The model under review builds one solid part; all positions refer to its coordinate system, in mm. Face numbers are marked on the shaded views. A direction names the side the tool comes from. Round coordinates to 2 decimals unless told otherwise and drop trailing zeros. Loops run counter-clockwise (first coordinate to the right, second up) from the corner with the lowest first, then second, coordinate; pieces in that order, holes last. Notation, with made-up numbers: (71, 57.25) -> (125, 57.25) arc R12 ccw to (125, 67.25) -> close; hole circle Ø6 at (37.5, 74.5). An arc over 180 degrees is marked (long way). Write each question's results on one line, items separated by ' | '. Start each with the question number.
Item 1: Clearance check with flat-ended pins moving along their axes: pin 1 Ø6 at (x, z) = (39, 6.5) entering from -Y; pin 2 Ø1.5 at (x, z) = (39.5, 7) entering from -Y; pin 3 Ø6 at (x, y) = (31.5, -16.5) entering from +Z. State where each tip first meets the part, or that it passes through.
Item 2: Tool access review of the marked faces 1, 2 and 3: name each direction out of +Z, -Z, +X, -X, +Y, -Y from which nothing blocks a thin tool from reaching the whole face with its end or side.
Item 3: We need section C-C (y = -39.13). Give the boundary of the cut face in (x, z), and give its area (3 significant figures).
Item 4: For L1, parallel to Y at x = 25.25, z = 6.1; L2, parallel to X at y = 16, z = 9; L3, parallel to Y at x = 30.87, z = 2.85, list the stretches that pass through material, from the lowest coordinate up. Write a range as from..to.
Item 5: Mouldability with a two-part tool opening along X and no side actions: class the marked faces 4, 5, 6 and 7 as pulls with the +X half, pulls with the -X half, needs draft (parallel to the pull), parting line crosses it, or undercut.
Item 6: We need section D-D (y = -24.13). Give the boundary of the cut face in (x, z).
Item 7: We need section B-B (z = 3.25). Give the boundary of the cut face in (x, y), and give its area (3 significant figures).
Item 8: We need section A-A (y = 24.13). Give the boundary of the cut face in (x, z).
from build123d import *

# Parameters (mm, degrees)
SKETCH_W     = 20
SKETCH_H     = 83.26
SKETCH_R     = 1.75
SKETCH_R_2   = 2.25
PAD_DEPTH    = 5
PAD001_DEPTH = 5


with BuildPart() as part:
    # Sketch → Pad (new body)
    with BuildSketch(Plane.XY):
        with Locations((30.87, -7.5)):
            Rectangle(SKETCH_W, SKETCH_H)
        with Locations((25.25, -24.13)):
            Circle(SKETCH_R, mode=Mode.SUBTRACT)
        with Locations((32.87, 24.13)):
            Circle(SKETCH_R, mode=Mode.SUBTRACT)
        with Locations((30.87, -39.13)):
            Circle(SKETCH_R_2, mode=Mode.SUBTRACT)
    extrude(amount=PAD_DEPTH)

    # Sketch001 → Pad001 (new body)
    with BuildSketch(Plane.XY.offset(5)):
        with BuildLine():
            Line((20.87, 34.13), (20.87, -29.13))
            Line((20.87, -29.13), (25.87, -29.13))
            Line((25.87, -29.13), (25.87, -28.081658))
            ThreePointArc((25.87, -20.178342), (21.25, -24.13), (25.87, -28.081658))
            Line((25.87, 34.13), (25.87, -20.178342))
            Line((20.87, 34.13), (25.87, 34.13))
        make_face()
        with BuildLine():
            Line((40.87, 34.13), (35.87, 34.13))
            Line((35.87, 34.13), (35.87, 26.775751))
            ThreePointArc((35.87, 21.484249), (36.87, 24.13), (35.87, 26.775751))
            Line((35.87, -29.13), (35.87, 21.484249))
            Line((35.87, -29.13), (40.87, -29.13))
            Line((40.87, -29.13), (40.87, 34.13))
        make_face()
    extrude(amount=PAD001_DEPTH)


solid = part.part
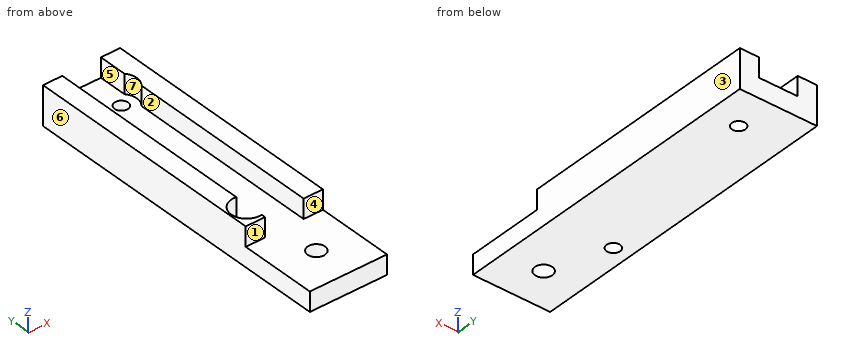
Here are the results:
1) pin 1: stops at y = -49.13 | pin 2: stops at y = -29.13 | pin 3: stops at z = 5
2) face 1: +Z, +X, -X, -Y | face 2: +Z, +Y, -Y | face 3: +Z, -Z, +X, +Y, -Y
3) outline: (20.87, 0) -> (28.62, 0) -> (28.62, 5) -> (20.87, 5) -> close; (33.12, 0) -> (40.87, 0) -> (40.87, 5) -> (33.12, 5) -> close | area: 77.5 mm2
4) L1: y = -29.13..-28.13, -20.13..34.13 | L2: x = 20.87..25.87, 35.87..40.87 | L3: y = -49.13..-41.38, -36.88..34.13
5) face 4: needs draft | face 5: undercut | face 6: pulls with the -X half | face 7: undercut
6) outline: (20.87, 0) -> (23.5, 0) -> (23.5, 5) -> (21.25, 5) -> (21.25, 10) -> (20.87, 10) -> close; (27, 0) -> (40.87, 0) -> (40.87, 10) -> (35.87, 10) -> (35.87, 5) -> (27, 5) -> close
7) outline: (20.87, -49.13) -> (40.87, -49.13) -> (40.87, 34.13) -> (20.87, 34.13) -> close; hole circle Ø3.5 at (25.25, -24.13); hole circle Ø4.5 at (30.87, -39.13); hole circle Ø3.5 at (32.87, 24.13) | area: 1,630 mm2
8) outline: (20.87, 0) -> (31.12, 0) -> (31.12, 5) -> (25.87, 5) -> (25.87, 10) -> (20.87, 10) -> close; (34.62, 0) -> (40.87, 0) -> (40.87, 10) -> (36.87, 10) -> (36.87, 5) -> (34.62, 5) -> close
